```python
from build123d import *

# Parameters (mm, degrees)
EXTRUDE_1_DEPTH     = 15
SKETCH_2_R          = 1.1
SKETCH_2_R_2        = 2.02
CUT_EXTRUDE_1_DEPTH = 15
CUT_EXTRUDE_2_REACH = 125.786
FILLET_1_R          = 10


with BuildPart() as part:
    # 草图1 → 凸台-拉伸1 (new body)
    with BuildSketch(Plane(origin=(0, 0, 0), x_dir=(1, 0, 0), z_dir=(0, 1, 0))):
        with BuildLine():
            Line((0, 0), (60, 0))
            add(Edge.make_bspline(
                [(60, 0), (115, -5), (120, -15)],
                knots=[0, 0, 0, 1, 1, 1], degree=2))
            Line((120, -15), (85, -15))
            ThreePointArc((85, -15), (81, -13), (77, -15))
            Line((77, -15), (70, -15))
            ThreePointArc((70, -15), (62.5, -10.974937186), (55, -15))
            Line((55, -15), (48, -15))
            ThreePointArc((48, -15), (28.349696115, -6.013929798), (7.758330249, -12.562177826))
            Line((7.758330249, -12.562177826), (-0.241669751, -26.418584287))
            Line((-0.241669751, -26.418584287), (-11.5, -19.918584287))
            Line((-11.5, -19.918584287), (0, 0))
        make_face()
    extrude(amount=EXTRUDE_1_DEPTH)

    # 草图2 → 切除-拉伸1 (cut)
    with BuildSketch(Plane(origin=(0, 15, 0), x_dir=(1, 0, 0), z_dir=(0, 1, 0))):
        with Locations(Location((5, -3, 0), (0, 0, 270))):
            Circle(SKETCH_2_R)
        with Locations(Location((30, -3, 0), (0, 0, 270))):
            Circle(SKETCH_2_R)
        with Locations(Location((55, -3, 0), (0, 0, 270))):
            Circle(SKETCH_2_R)
        with Locations(Location((60, -3, 0), (0, 0, 270))):
            Circle(SKETCH_2_R)
        with Locations(Location((45, -8, 0), (0, 0, 270))):
            Circle(SKETCH_2_R)
        with Locations(Location((50, -8, 0), (0, 0, 270))):
            Circle(SKETCH_2_R)
        with Locations(Location((55, -8, 0), (0, 0, 270))):
            Circle(SKETCH_2_R)
        with Locations(Location((60, -8, 0), (0, 0, 270))):
            Circle(SKETCH_2_R)
        with Locations(Location((65, -3, 0), (0, 0, 270))):
            Circle(SKETCH_2_R)
        with Locations(Location((65, -8, 0), (0, 0, 270))):
            Circle(SKETCH_2_R)
        with Locations(Location((70, -8, 0), (0, 0, 270))):
            Circle(SKETCH_2_R)
        with Locations(Location((75, -8, 0), (0, 0, 270))):
            Circle(SKETCH_2_R)
        with Locations(Location((70, -3, 0), (0, 0, 270))):
            Circle(SKETCH_2_R)
        with Locations(Location((-4.303847577, -19.454482672, 0), (0, 0, 270))):
            Circle(SKETCH_2_R_2)
        with Locations(Location((50, -3, 0), (0, 0, 270))):
            Circle(SKETCH_2_R)
        with Locations(Location((-0.303847577, -12.526279442, 0), (0, 0, 270))):
            Circle(SKETCH_2_R_2)
        with Locations(Location((80, -8, 0), (0, 0, 270))):
            Circle(SKETCH_2_R)
        with Locations(Location((85, -8, 0), (0, 0, 270))):
            Circle(SKETCH_2_R)
        with Locations(Location((90, -8, 0), (0, 0, 270))):
            Circle(SKETCH_2_R)
        with Locations(Location((95, -8, 0), (0, 0, 270))):
            Circle(SKETCH_2_R)
        with Locations(Location((100, -8, 0), (0, 0, 270))):
            Circle(SKETCH_2_R)
        with BuildLine():
            Line((10, -4.1), (25, -4.1))
            ThreePointArc((25, -4.1), (26.1, -3), (25, -1.9))
            Line((25, -1.9), (10, -1.9))
            ThreePointArc((10, -1.9), (8.9, -3), (10, -4.1))
        make_face()
        with BuildLine():
            Line((35, -1.9), (45, -1.9))
            ThreePointArc((45, -1.9), (46.1, -3), (45, -4.1))
            Line((45, -4.1), (35, -4.1))
            ThreePointArc((35, -4.1), (33.9, -3), (35, -1.9))
        make_face()
        with BuildLine():
            Line((5, -6.9), (10, -6.9))
            ThreePointArc((10, -6.9), (11.1, -8), (10, -9.1))
            Line((10, -9.1), (5, -9.1))
            ThreePointArc((5, -9.1), (3.9, -8), (5, -6.9))
        make_face()
    extrude(amount=-CUT_EXTRUDE_1_DEPTH, mode=Mode.SUBTRACT)

    # 草图4 → 切除-拉伸2 (cut, up to next)
    with BuildSketch(Plane(origin=(0, 15, 0), x_dir=(1, 0, 0), z_dir=(0, 1, 0)), mode=Mode.PRIVATE) as cut_extrude_2_sk1:
        Polygon((85, -15), (115.991250003, -11.194752977), (120, -11.194752977), (120, -15), align=None)
    cut_extrude_2_tool1 = extrude(cut_extrude_2_sk1.sketch, amount=-CUT_EXTRUDE_2_REACH, mode=Mode.PRIVATE) & part.part
    add(cut_extrude_2_tool1.solids().sort_by_distance((108.196013, 15, 13.601235))[0], mode=Mode.SUBTRACT)

    # 圆角1
    fillet_1_edges = [part.edges().sort_by_distance(p)[0] for p in [
        (0, 7.5, 0),
    ]]
    fillet(fillet_1_edges, radius=FILLET_1_R)


solid = part.part
```
Can you work these out from the model? Positions are in its coordinate system, mm. A direction names the side the tool comes from. Give positions to 0.01 mm unless a question says otherwise; leave off trailing zeros. Order: outer loops, then holes, each group sorted by start corner. A loop starts at its lowest first (then second) coordinate and runs counter-clockwise, first axis right, second up. Notation, with made-up numbers: M 22,66.5 L 39,66.5 A23 ccw 39,98.5 Z; hole C 48,53 d2. An arc over 180 degrees is marked long. One line per item, written item: value.
1) I want a section at D-D, the plane x = 37. List the corners of the cut face in (y, z) for me, plus the area to 3 significant figures.
Answer sheet:
outline: M 0,0 L 15,0 L 15,1.9 L 0,1.9 Z; M 0,4.1 L 15,4.1 L 15,7.84 L 0,7.84 Z
area: 84.6 mm^2
2) For P1, Ø8, axis at x = 9.5, y = 9, coming from the +Z side; P2, Ø4.5, axis at x = 15.5, y = 8, coming from the +Z side; P3, Ø4.5, axis at x = -4.3, z = 19.45, coming from the -Y side; P4, Ø1.3, axis at x = 70, z = 8, coming from the +Y side, each with a flat end and sliding along its axis, tell me the tip position at first contact or that it passes through.
Answer sheet:
P1: stops at z = 16.47
P2: stops at z = 9.06
P3: stops at y = 0
P4: passes through
3) Please list where these lines run through material, in increasing order: line 1 along Z through (x, y) = (64, 13.75); line 2 along Z through (x, y) = (26, 2.5); line 3 along Z through (x, y) = (23, 1.25).
Answer sheet:
line 1: z = 0.38 to 2.54, 3.46 to 7.54, 8.46 to 11.1
line 2: z = 0 to 2.54, 3.46 to 5.96
line 3: z = 0 to 1.9, 4.1 to 6.17
4) I want a section at C-C, the plane y = 4.5. Count the separate pieces of the cut face and the enclosed holes in it, plus the area to 3 significant figures.
Answer sheet:
separate pieces: 1
enclosed holes: 24
area: 1,140 mm^2
5) I want a section at B-B, the plane x = 20.5. List the corners of the cut face in (y, z) for me.
Answer sheet:
outline: M 0,0 L 15,0 L 15,1.9 L 0,1.9 Z; M 0,4.1 L 15,4.1 L 15,6.57 L 0,6.57 Z
6) On a 3-axis mill with a long thin cutter (end or side, diameter ignored), from which of +Z, -Z, +X, -X, +Y, -Y can I reach the whole of each face in a straight line? I mean faces 1 (the face through (-7.25, 7.4, 12.56)), 2 (the face through (52, 7, 15)), 3 (the face through (3.814, 7.395, 19.393)), 4 (the face through (17, 8, 4.1)). Say none if no direction works.
Answer sheet:
face 1: -Z, -X, +Y, -Y
face 2: +Z, +X, +Y, -Y
face 3: +Z, +Y, -Y
face 4: +Y, -Y
7) We'd pull the mould along X, two halves only. Please class faces 5 (the face through (-4.215, 7.605, 17.436)), 6 (the face through (50.93, 7.6, 8.59)), 7 (the face through (48, 15, 8)), 8 (the face through (0.84, 7.6, 1.3)): released by +X, released by -X, zero draft, split by the parting line, or undercut.
Answer sheet:
face 5: undercut
face 6: undercut
face 7: zero draft
face 8: released by -X
8) I want a section at A-A, the plane x = 50. List the corners of the cut face in (y, z) for me.
Answer sheet:
outline: M 0,0 L 15,0 L 15,1.9 L 0,1.9 Z; M 0,4.1 L 15,4.1 L 15,6.9 L 0,6.9 Z; M 0,9.1 L 15,9.1 L 15,15 L 0,15 Z
